```python
from build123d import *

# Parameters (mm, degrees)
SKETCH1_W           = 132
SKETCH1_H           = 98
BOSS_EXTRUDE1_DEPTH = 55
FILLET1_R           = 14
SKETCH7_R           = 6
BOSS_EXTRUDE2_DEPTH = 6
SKETCH8_R           = 2.25
CUT_EXTRUDE10_DEPTH = 6.2
SKETCH9_R           = 4
CUT_EXTRUDE11_DEPTH = 3
FILLET2_R           = 3
SKETCH10_W          = 44
SKETCH10_H          = 44
BOSS_EXTRUDE3_DEPTH = 8
FILLET3_R           = 5
FILLET4_R           = 1.5
SKETCH11_R          = 2.15
BOSS_EXTRUDE4_DEPTH = 11.8
SKETCH12_R          = 0.75
CUT_EXTRUDE12_DEPTH = 11.3
SKETCH13_R          = 5
CUT_EXTRUDE13_DEPTH = 3.2
FILLET5_R           = 3
SKETCH14_W          = 104
SKETCH14_H          = 92
CUT_EXTRUDE14_DEPTH = 52.6
SKETCH15_W          = 126
SKETCH15_H          = 70
CUT_EXTRUDE15_DEPTH = 52.6
SKETCH17_R          = 6.2
BOSS_EXTRUDE5_DEPTH = 6
SKETCH18_R          = 2.25
CUT_EXTRUDE17_DEPTH = 6.2
SKETCH19_R          = 4
CUT_EXTRUDE18_DEPTH = 3


with BuildPart() as part:
    # Sketch1 → Boss-Extrude1 (new body)
    with BuildSketch(Plane.XY):
        Rectangle(SKETCH1_W, SKETCH1_H)
    extrude(amount=BOSS_EXTRUDE1_DEPTH)

    # Fillet1
    fillet1_edges = [part.edges().sort_by_distance(p)[0] for p in [
        (-66, 49, 27.5),
        (66, 49, 27.5),
        (66, -49, 27.5),
        (-66, -49, 27.5),
    ]]
    fillet(fillet1_edges, radius=FILLET1_R)

    # Sketch7 → Boss-Extrude2 (add)
    with BuildSketch(Plane.XY):
        with Locations((-27.75, -42.789)):
            Circle(SKETCH7_R)
        with Locations((27.75, -42.789)):
            Circle(SKETCH7_R)
        with Locations((-27.75, 42.789)):
            Circle(SKETCH7_R)
        with Locations((27.75, 42.789)):
            Circle(SKETCH7_R)
    extrude(amount=BOSS_EXTRUDE2_DEPTH)

    # Sketch8 → Cut-Extrude10 (cut)
    with BuildSketch(Plane.XY.offset(6)):
        with Locations((-27.75, -42.789)):
            Circle(SKETCH8_R)
        with Locations((27.75, -42.789)):
            Circle(SKETCH8_R)
        with Locations((-27.75, 42.789)):
            Circle(SKETCH8_R)
        with Locations((27.75, 42.789)):
            Circle(SKETCH8_R)
    extrude(amount=-CUT_EXTRUDE10_DEPTH, mode=Mode.SUBTRACT)

    # Sketch9 → Cut-Extrude11 (cut)
    with BuildSketch(Plane.XY.offset(6)):
        with Locations((-27.75, -42.789)):
            Circle(SKETCH9_R)
        with Locations((27.75, -42.789)):
            Circle(SKETCH9_R)
        with Locations((-27.75, 42.789)):
            Circle(SKETCH9_R)
        with Locations((27.75, 42.789)):
            Circle(SKETCH9_R)
    extrude(amount=-CUT_EXTRUDE11_DEPTH, mode=Mode.SUBTRACT)

    # Fillet2
    fillet2_edges = [part.edges().sort_by_distance(p)[0] for p in [
        (-66, 0, 55),
        (0, 49, 55),
        (0, -49, 55),
        (66, 0, 55),
        (-61.899494937, -44.899494937, 55),
        (61.899494937, -44.899494937, 55),
        (61.899494937, 44.899494937, 55),
        (-61.899494937, 44.899494937, 55),
    ]]
    fillet(fillet2_edges, radius=FILLET2_R)

    # Sketch10 → Boss-Extrude3 (add)
    with BuildSketch(Plane.XY.offset(55)):
        Rectangle(SKETCH10_W, SKETCH10_H)
    extrude(amount=BOSS_EXTRUDE3_DEPTH)

    # Fillet3
    fillet3_edges = [part.edges().sort_by_distance(p)[0] for p in [
        (-22, 22, 59),
        (-22, -22, 59),
        (22, -22, 59),
        (22, 22, 59),
    ]]
    fillet(fillet3_edges, radius=FILLET3_R)

    # Fillet4
    fillet4_edges = [part.edges().sort_by_distance(p)[0] for p in [
        (-22, 0, 63),
        (0, 22, 63),
        (0, -22, 63),
        (22, 0, 63),
        (-20.535533906, -20.535533906, 63),
        (20.535533906, -20.535533906, 63),
        (20.535533906, 20.535533906, 63),
        (-20.535533906, 20.535533906, 63),
    ]]
    fillet(fillet4_edges, radius=FILLET4_R)

    # Sketch11 → Boss-Extrude4 (add)
    with BuildSketch(Plane.XY.offset(63)):
        with Locations(Location((-14.1, 14.1, 0), (0, 0, 180))):
            Circle(SKETCH11_R)
        with Locations(Location((14.1, -14.1, 0), (0, 0, 180))):
            Circle(SKETCH11_R)
    extrude(amount=BOSS_EXTRUDE4_DEPTH)

    # Sketch12 → Cut-Extrude12 (cut)
    with BuildSketch(Plane.XY.offset(74.8)):
        with Locations((-14.1, 14.1)):
            Circle(SKETCH12_R)
        with Locations((14.1, -14.1)):
            Circle(SKETCH12_R)
    extrude(amount=-CUT_EXTRUDE12_DEPTH, mode=Mode.SUBTRACT)

    # Sketch13 → Cut-Extrude13 (cut)
    with BuildSketch(Plane.XY.offset(55)):
        with Locations((-40, -37)):
            Circle(SKETCH13_R)
        with Locations((40, -37)):
            Circle(SKETCH13_R)
        with Locations((0, -35)):
            Circle(SKETCH13_R)
    extrude(amount=-CUT_EXTRUDE13_DEPTH, mode=Mode.SUBTRACT)

    # Fillet5
    fillet5_edges = [part.edges().sort_by_distance(p)[0] for p in [
        (-22, 0, 55),
        (0, 22, 55),
        (22, 0, 55),
        (0, -22, 55),
        (-20.535533906, 20.535533906, 55),
        (20.535533906, 20.535533906, 55),
        (20.535533906, -20.535533906, 55),
        (-20.535533906, -20.535533906, 55),
    ]]
    fillet(fillet5_edges, radius=FILLET5_R)

    # Sketch14 → Cut-Extrude14 (cut)
    with BuildSketch(Plane(origin=(0, 0, 0), x_dir=(-1, 0, 0), z_dir=(0, 0, -1))):
        Rectangle(SKETCH14_W, SKETCH14_H)
    extrude(amount=-CUT_EXTRUDE14_DEPTH, mode=Mode.SUBTRACT)

    # Sketch15 → Cut-Extrude15 (cut)
    with BuildSketch(Plane(origin=(0, 0, 0), x_dir=(-1, 0, 0), z_dir=(0, 0, -1))):
        Rectangle(SKETCH15_W, SKETCH15_H)
    extrude(amount=-CUT_EXTRUDE15_DEPTH, mode=Mode.SUBTRACT)

    # Sketch17 → Boss-Extrude5 (add)
    with BuildSketch(Plane.XY):
        with Locations((-27.75, -42.789)):
            Circle(SKETCH17_R)
        with Locations((27.75, -42.789)):
            Circle(SKETCH17_R)
        with Locations((-27.75, 42.789)):
            Circle(SKETCH17_R)
        with Locations((27.75, 42.789)):
            Circle(SKETCH17_R)
    extrude(amount=BOSS_EXTRUDE5_DEPTH)

    # Sketch18 → Cut-Extrude17 (cut)
    with BuildSketch(Plane.XY.offset(6)):
        with Locations((-27.75, -42.789)):
            Circle(SKETCH18_R)
        with Locations((27.75, -42.789)):
            Circle(SKETCH18_R)
        with Locations((-27.75, 42.789)):
            Circle(SKETCH18_R)
        with Locations((27.75, 42.789)):
            Circle(SKETCH18_R)
    extrude(amount=-CUT_EXTRUDE17_DEPTH, mode=Mode.SUBTRACT)

    # Sketch19 → Cut-Extrude18 (cut)
    with BuildSketch(Plane.XY.offset(6)):
        with Locations((-27.75, -42.789)):
            Circle(SKETCH19_R)
        with Locations((27.75, -42.789)):
            Circle(SKETCH19_R)
        with Locations((-27.75, 42.789)):
            Circle(SKETCH19_R)
        with Locations((27.75, 42.789)):
            Circle(SKETCH19_R)
    extrude(amount=-CUT_EXTRUDE18_DEPTH, mode=Mode.SUBTRACT)


solid = part.part
```
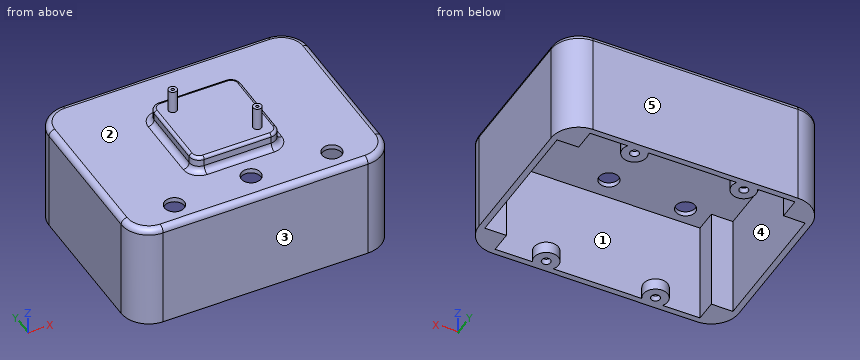
Part model, mm, in its own coordinate system. Face numbers are marked on the shaded views. A direction names the side the tool comes from. Coordinates: 2 decimals unless noted, no trailing zeros. Order: outer loops, then holes, each group sorted by start corner. A loop starts at its lowest first (then second) coordinate and runs counter-clockwise, first axis right, second up. Notation, with made-up numbers: (49.5, 9.25) -> (98.5, 9.25) arc R26 cw to (98.5, 29.25) -> close; hole circle Ø1 at (85, 46.5). An arc over 180 degrees is marked (long way). Put each result on its own line as item: value. Start each with the question number.
(1) Band-saw the part on C-C (x = -27.75). Count the separate pieces of the cut face and the enclosed holes in it, then the cut area to 3 significant figures.
(2) Band-saw the part on A-A (x = 0). Give the cut face in (y, z), then the cut area to 3 significant figures.
(3) Band-saw the part on D-D (z = 70). Give the cut face in (x, y).
(4) Band-saw the part on B-B (z = 47). Give the cut face in (x, y), then the cut area to 3 significant figures.
(5) Probe line 1 along Y through (x, z) = (27.75, 0.85); line 2 along X through (y, z) = (-19, 33.5); line 3 along X through (y, z) = (14, 67). List the from-to ranges inside material, lowest first. Write a range as [from, to].
(6) Mould opens along Y. For the marked faces 1, 2 and 3 say: pulls with the +Y half, pulls with the -Y half, needs draft (parallel to the pull), parting line crosses it, or undercut.
(7) Which spindle directions (+Z, -Z, +X, -X, +Y, -Y) get a long thin tool onto all of the face, cutting with end or side? Do the marked faces 4 and 5. Say none if no direction does.
(8) Pin check, flat tips, straight feed: pin 1 Ø4 at (x, y) = (2, 10.5) entering from -Z; pin 2 Ø4 at (x, y) = (-27, 42) entering from +Z; pin 3 Ø3.5 at (x, z) = (-56, 15.5) entering from -Y. Stop position of each tip, or through.
Determined:
1. separate pieces: 3
1. enclosed holes: 0
1. area: 585 mm²
2. outline: (-49, 0) -> (-46, 0) -> (-46, 52.6) -> (-40, 52.6) -> (-40, 55) -> (-46, 55) arc R3 ccw to (-49, 52) -> close; (-30, 52.6) -> (46, 52.6) -> (46, 0) -> (49, 0) -> (49, 52) arc R3 ccw to (46, 55) -> (25, 55) arc R3 cw to (22, 58) -> (22, 61.5) arc R1.5 ccw to (20.5, 63) -> (-20.5, 63) arc R1.5 ccw to (-22, 61.5) -> (-22, 58) arc R3 cw to (-25, 55) -> (-30, 55) -> close
2. area: 878 mm²
3. outline: circle Ø4.3 at (-14.1, 14.1); circle Ø4.3 at (14.1, -14.1); hole circle Ø1.5 at (-14.1, 14.1); hole circle Ø1.5 at (14.1, -14.1)
4. outline: (-66, -35) arc R14 ccw to (-52, -49) -> (52, -49) arc R14 ccw to (66, -35) -> (66, 35) arc R14 ccw to (52, 49) -> (-52, 49) arc R14 ccw to (-66, 35) -> close; hole (-63, -35) -> (-52, -35) -> (-52, -46) -> (52, -46) -> (52, -35) -> (63, -35) -> (63, 35) -> (52, 35) -> (52, 46) -> (-52, 46) -> (-52, 35) -> (-63, 35) -> close
4. area: 1,660 mm²
5. line 1: y = [-49, -45.04], [-40.54, -36.59], [36.59, 40.54], [45.04, 49]
5. line 2: x = [-66, -63], [63, 66]
5. line 3: x = [-16.25, -14.84], [-13.36, -11.95]
6. face 1: undercut
6. face 2: needs draft
6. face 3: pulls with the -Y half
7. face 4: -Z
7. face 5: +Z, -Z, +X, -X, +Y
8. pin 1: stops at z = 52.6
8. pin 2: stops at z = 55
8. pin 3: stops at y = -48.82
